from build123d import *

# Parameters (mm, degrees)
SKETCH1_R           = 2.5
BOSS_EXTRUDE1_DEPTH = 100
CUT_EXTRUDE1_DEPTH  = 5
BOSS_EXTRUDE2_DEPTH = 1
CUT_EXTRUDE2_DEPTH  = 6
CHAMFER1_SIZE       = 1


with BuildPart() as part:
    # Sketch1 → Boss-Extrude1 (new body)
    with BuildSketch(Plane.XY):
        Circle(SKETCH1_R)
    extrude(amount=BOSS_EXTRUDE1_DEPTH)

    # Sketch2 → Cut-Extrude1 (cut, symmetric)
    with BuildSketch(Plane(origin=(0, 0, 0), x_dir=(0, 0, -1), z_dir=(1, 0, 0))):
        with BuildLine():
            Line((-94, 4), (-88, 4))
            ThreePointArc((-88, 4), (-87.292893219, 3.707106781), (-87, 3))
            Line((-87, 3), (-87, 2))
            ThreePointArc((-87, 2), (-87.292893219, 1.292893219), (-88, 1))
            Line((-88, 1), (-94, 1))
            ThreePointArc((-94, 1), (-94.707106781, 1.292893219), (-95, 2))
            Line((-95, 2), (-95, 3))
            ThreePointArc((-95, 3), (-94.707106781, 3.707106781), (-94, 4))
        make_face()
        with BuildLine():
            Line((-87, -3), (-87, -2))
            ThreePointArc((-87, -2), (-87.292893219, -1.292893219), (-88, -1))
            Line((-88, -1), (-94, -1))
            ThreePointArc((-94, -1), (-94.707106781, -1.292893219), (-95, -2))
            Line((-95, -2), (-95, -3))
            ThreePointArc((-95, -3), (-94.707106781, -3.707106781), (-94, -4))
            Line((-94, -4), (-88, -4))
            ThreePointArc((-88, -4), (-87.292893219, -3.707106781), (-87, -3))
        make_face()
    extrude(amount=CUT_EXTRUDE1_DEPTH, both=True, mode=Mode.SUBTRACT)

    # Sketch2<2> → Boss-Extrude2 (add, symmetric)
    with BuildSketch(Plane(origin=(0, 0, 0), x_dir=(0, 0, -1), z_dir=(1, 0, 0))):
        with BuildLine():
            Line((-94, 4), (-88, 4))
            ThreePointArc((-88, 4), (-87.292893219, 3.707106781), (-87, 3))
            Line((-87, 3), (-87, 2))
            ThreePointArc((-87, 2), (-87.292893219, 1.292893219), (-88, 1))
            Line((-88, 1), (-94, 1))
            ThreePointArc((-94, 1), (-94.707106781, 1.292893219), (-95, 2))
            Line((-95, 2), (-95, 3))
            ThreePointArc((-95, 3), (-94.707106781, 3.707106781), (-94, 4))
        make_face()
        with BuildLine():
            Line((-87, -3), (-87, -2))
            ThreePointArc((-87, -2), (-87.292893219, -1.292893219), (-88, -1))
            Line((-88, -1), (-94, -1))
            ThreePointArc((-94, -1), (-94.707106781, -1.292893219), (-95, -2))
            Line((-95, -2), (-95, -3))
            ThreePointArc((-95, -3), (-94.707106781, -3.707106781), (-94, -4))
            Line((-94, -4), (-88, -4))
            ThreePointArc((-88, -4), (-87.292893219, -3.707106781), (-87, -3))
        make_face()
    extrude(amount=BOSS_EXTRUDE2_DEPTH, both=True)

    # Sketch4 → Cut-Extrude2 (cut, symmetric)
    with BuildSketch(Plane(origin=(0, 0, 0), x_dir=(0, 0, -1), z_dir=(1, 0, 0))):
        Polygon((-15, 2.5), (0, 1), (0, 2.5), align=None)
        Polygon((0, -2.5), (0, -1), (-15, -2.5), align=None)
    extrude(amount=CUT_EXTRUDE2_DEPTH, both=True, mode=Mode.SUBTRACT)

    # Chamfer1
    chamfer1_edges = [part.edges().sort_by_distance(p)[0] for p in [
        (-2.5, 0, 100),
    ]]
    chamfer(chamfer1_edges, length=CHAMFER1_SIZE)


solid = part.part
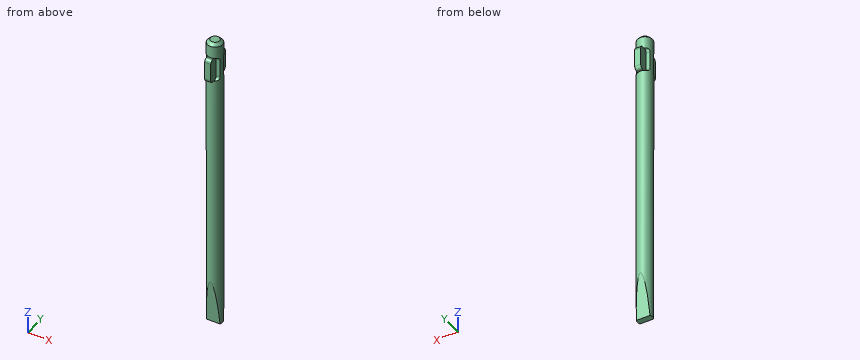
Can you work these out from the model? Positions are in its coordinate system, mm. Coordinates: 2 decimals unless noted, no trailing zeros. Write each loop counter-clockwise with the first axis right and the second up, starting at its lowest first coordinate (ties: lowest second). Pieces come first, ordered by that corner, then holes. Notation, with made-up numbers: (77, 30) - (121, 30) arc R13 ccw to (121, 45) - close; hole circle Ø9 at (18, 52.5). An arc over 180 degrees is marked (long way). Return JSON: item names as keys, results as strings. Group by question number.
Item 1: I'm going to push flat-ended pins straight in: pin 1 Ø1.5 at (x, y) = (1, -2.5) entering from +Z; pin 2 Ø0.8 at (x, y) = (0, 2.5) entering from +Z; pin 3 Ø0.9 at (y, z) = (2.5, 90.5) entering from -X. Where does each tip first touch, or does it pass through?
Item 2: If we section it at A-A (x = 0): Write out the boundary of the cut face in (y, z).
Item 3: If we section it at B-B (z = 26.5): Write out the boundary of the cut face in (x, y), then the cut area to 3 significant figures.
Item 4: Please list where these lines run through material, in increasing order: probe 1 along Y at (x, z) = (0.2, 38); probe 2 along Y at (x, z) = (-1.5, 36); probe 3 along X at (y, z) = (1, 36).
Item 5: If we section it at C-C (z = 12): Write out the boundary of the cut face in (x, y).
Return value:
{
 "1": {"pin 1": "stops at z = 99.56", "pin 2": "stops at z = 99.4", "pin 3": "stops at x = -1"},
 "2": {"outline": "(-4, 88) arc R1 ccw to (-3, 87) - (-2.5, 87) - (-2.5, 15) - (-1, 0) - (1, 0) - (2.5, 15) - (2.5, 87) - (3, 87) arc R1 ccw to (4, 88) - (4, 94) arc R1 ccw to (3, 95) - (2.5, 95) - (2.5, 99) - (1.5, 100) - (-1.5, 100) - (-2.5, 99) - (-2.5, 95) - (-3, 95) arc R1 ccw to (-4, 94) - close"},
 "3": {"outline": "circle Ø5 at (0, 0)", "area": "19.6 mm^2"},
 "4": {"probe 1": "y = -2.49 to 2.49", "probe 2": "y = -2 to 2", "probe 3": "x = -2.29 to 2.29"},
 "5": {"outline": "(-1.19, -2.2) - (1.19, -2.2) arc R2.5 ccw to (1.19, 2.2) - (-1.19, 2.2) arc R2.5 ccw to start"}
}
